```python
from build123d import *

# Parameters (mm, degrees)
F1_DEPTH = 10
F2_R     = 1.55
F3_DEPTH = 1.2


with BuildPart() as f1:
    # F0 (on Top) → F1 (new body)
    with BuildSketch(Plane.XY):
        Polygon((23.076923, 0), (-5.723077, 0), (-5.723077, -1.2), (24.276923, -1.2), (24.276923, 13.8), (23.076923, 13.8), align=None)
    extrude(amount=F1_DEPTH)

    # F2 (on face) → F3 (cut)
    with BuildSketch(Plane.YZ.offset(24.276923)):
        with Locations((6, 5)):
            Circle(F2_R)
    extrude(amount=-F3_DEPTH, mode=Mode.SUBTRACT)


solid = f1.part
```
Work out the finished part from the listing and answer in its coordinate system (mm). A direction names the side the tool comes from. Round coordinates to 2 decimals unless told otherwise and drop trailing zeros. Order: outer loops, then holes, each group sorted by start corner. A loop starts at its lowest first (then second) coordinate and runs counter-clockwise, first axis right, second up.
Q1. Find the intervals of material crossed by line 1 along Z through (x, y) = (23.5, 6); line 2 along X through (y, z) = (0.5, 6.25); line 3 along Y through (x, z) = (-3.75, 7.25), in increasing order.
Solution:
line 1: z = 0 to 3.45, 6.55 to 10
line 2: x = 23.08 to 24.28
line 3: y = -1.2 to 0
Q2. The mould has two halves that part along Y. Classify faces 3 (the flat face through (13.7, -0.3, 10)), 4 (the flat face through (9, -1.2, 5)), 5 (the cylindrical face through (23.69, 4.45, 5.07)): pulls with the +Y half, pulls with the -Y half, needs draft (parallel to the pull), parting line crosses it, or undercut.
Solution:
face 3: needs draft
face 4: pulls with the -Y half
face 5: undercut
Q3. A tool of negligible diameter and unlimited length cuts with its end or side. For faces 1 (the flat face through (23.077, 9, 5)), 2 (the flat face through (24, 13.8, 5)), from which of +Z, -Z, +X, -X, +Y, -Y can it reach the whole face along a straight path? Write none if from no direction.
Solution:
face 1: +Z, -Z, -X, +Y
face 2: +Z, -Z, +X, -X, +Y
Q4. A cutting plane is placed at C-C, the plane x = 5.5. Determine the outline of the cut face in (y, z).
Solution:
outline: (-1.2, 0) - (0, 0) - (0, 10) - (-1.2, 10) - close
Q5. A cutting plane is placed at A-A, the plane y = 6. Determine the outline of the cut face in (x, z).
Solution:
outline: (23.08, 0) - (24.28, 0) - (24.28, 3.45) - (23.08, 3.45) - close; (23.08, 6.55) - (24.28, 6.55) - (24.28, 10) - (23.08, 10) - close
Q6. A cutting plane is placed at D-D, the plane z = 1.5. Determine the outline of the cut face in (x, y).
Solution:
outline: (-5.72, -1.2) - (24.28, -1.2) - (24.28, 13.8) - (23.08, 13.8) - (23.08, 0) - (-5.72, 0) - close
Q7. Given pin 1 Ø5 at (y, z) = (10, 6) entering from -X; pin 2 Ø4 at (y, z) = (5, 5) entering from +X, each flat-ended and moving along its own axis, determine where each tip first touches the part or whether it passes through.
Solution:
pin 1: stops at x = 23.08
pin 2: stops at x = 24.28
Q8. A cutting plane is placed at B-B, the plane z = 5. Determine the outline of the cut face in (x, y), then the cut area to 3 significant figures.
Solution:
outline: (-5.72, -1.2) - (24.28, -1.2) - (24.28, 4.45) - (23.08, 4.45) - (23.08, 0) - (-5.72, 0) - close; (23.08, 7.55) - (24.28, 7.55) - (24.28, 13.8) - (23.08, 13.8) - close
area: 48.8 mm2
